Source: CAD feature listing. Evaluate the final solid. Frame: model axes, mm. A direction names the side the tool comes from. Round coordinates to 2 decimals unless told otherwise and drop trailing zeros. Order: outer loops, then holes, each group sorted by start corner. A loop starts at its lowest first (then second) coordinate and runs counter-clockwise, first axis right, second up. Notation, with made-up numbers: (25, 57.5) -> (51, 57.5) arc R21 cw to (51, 68.5) -> close; hole circle Ø1 at (-37, 50.5). An arc over 180 degrees is marked (long way). Answer as CSV lines item,"result".
from build123d import *

# Parameters (mm, degrees)
CYLINDER081_R     = 1.6
CYLINDER081_DEPTH = 1.5
CYLINDER082_R     = 4
CYLINDER082_DEPTH = 1.5
CYLINDER083_R     = 1.6
CYLINDER083_DEPTH = 1.5
CYLINDER084_R     = 4
CYLINDER084_DEPTH = 1.5
BOX207_W          = 14
BOX207_H          = 9
BOX207_DEPTH      = 1.5
BOX206_W          = 14
BOX206_H          = 9
BOX206_DEPTH      = 1.5
BOX205_W          = 36
BOX205_H          = 12
BOX205_DEPTH      = 1.5
FILLET050_R       = 2
CYLINDER080_R     = 1.6
CYLINDER080_DEPTH = 1.5
CYLINDER079_R     = 4
CYLINDER079_DEPTH = 1.5


with BuildPart() as cylinder162:
    # Cylinder081 → Cylinder081 (new body)
    with BuildSketch(Plane(origin=(70.25, 15, 8.3), x_dir=(1, 0, 0), z_dir=(0, 0, 1))):
        Circle(CYLINDER081_R)
    extrude(amount=CYLINDER081_DEPTH)


with BuildPart() as cut104:
    # Cylinder082 → Cylinder082 (new body)
    with BuildSketch(Plane(origin=(70.25, 15, 8.3), x_dir=(1, 0, 0), z_dir=(0, 0, 1))):
        Circle(CYLINDER082_R)
    extrude(amount=CYLINDER082_DEPTH)

    # Cut104: cut Cylinder162
    add(cylinder162.part, mode=Mode.SUBTRACT)


with BuildPart() as cylinder164:
    # Cylinder083 → Cylinder083 (new body)
    with BuildSketch(Plane(origin=(59.25, 32.25, 8.3), x_dir=(1, 0, 0), z_dir=(0, 0, 1))):
        Circle(CYLINDER083_R)
    extrude(amount=CYLINDER083_DEPTH)


with BuildPart() as cut105:
    # Cylinder084 → Cylinder084 (new body)
    with BuildSketch(Plane(origin=(59.25, 32.25, 8.3), x_dir=(1, 0, 0), z_dir=(0, 0, 1))):
        Circle(CYLINDER084_R)
    extrude(amount=CYLINDER084_DEPTH)

    # Cut105: cut Cylinder164
    add(cylinder164.part, mode=Mode.SUBTRACT)


with BuildPart() as cube196:
    # Box207 → Box207 (new body)
    with BuildSketch(Plane(origin=(61, 19.5, 8.3), x_dir=(1, 0, 0), z_dir=(0, 0, 1))):
        with Locations((7, 4.5)):
            Rectangle(BOX207_W, BOX207_H)
    extrude(amount=BOX207_DEPTH)


with BuildPart() as cube195:
    # Box206 → Box206 (new body)
    with BuildSketch(Plane(origin=(43.5, 19.5, 8.3), x_dir=(1, 0, 0), z_dir=(0, 0, 1))):
        with Locations((7, 4.5)):
            Rectangle(BOX206_W, BOX206_H)
    extrude(amount=BOX206_DEPTH)


with BuildPart() as fillet050:
    # Box205 → Box205 (new body)
    with BuildSketch(Plane(origin=(41, 18, 8.3), x_dir=(1, 0, 0), z_dir=(0, 0, 1))):
        with Locations((18, 6)):
            Rectangle(BOX205_W, BOX205_H)
    extrude(amount=BOX205_DEPTH)

    # Cut106: cut Cube195
    add(cube195.part, mode=Mode.SUBTRACT)

    # Cut107: cut Cube196
    add(cube196.part, mode=Mode.SUBTRACT)

    # Fillet050
    fillet050_edges = [fillet050.edges().sort_by_distance(p)[0] for p in [
        (41, 18, 9.05),
        (41, 30, 9.05),
        (77, 18, 9.05),
        (77, 30, 9.05),
    ]]
    fillet(fillet050_edges, radius=FILLET050_R)


with BuildPart() as cylinder161:
    # Cylinder080 → Cylinder080 (new body)
    with BuildSketch(Plane(origin=(47.75, 15, 8.3), x_dir=(1, 0, 0), z_dir=(0, 0, 1))):
        Circle(CYLINDER080_R)
    extrude(amount=CYLINDER080_DEPTH)


with BuildPart() as fusion064:
    # Cylinder079 → Cylinder079 (new body)
    with BuildSketch(Plane(origin=(47.75, 15, 8.3), x_dir=(1, 0, 0), z_dir=(0, 0, 1))):
        Circle(CYLINDER079_R)
    extrude(amount=CYLINDER079_DEPTH)

    # Cut103: cut Cylinder161
    add(cylinder161.part, mode=Mode.SUBTRACT)

    # Fusion064: union Cut104, Cut105, Fillet050
    add(cut104.part)
    add(cut105.part)
    add(fillet050.part)


solid = fusion064.part
1. Pin query (flat end, axial travel): pin 1 (0.8 mm diameter, centred on x = 68.5, z = 9, fed in from +Y). Return the tip coordinate at first contact, or that it passes through.
Results below:
pin 1,"y = 30"
2. Reachability of faces 1 (the flat face through (43.5, 24, 9)), 2 (the flat face through (41, 24, 9)) from +Z, -Z, +X, -X, +Y, -Y: full face, straight path, thin tool, end or side. Return the list, or none.
Results below:
face 1,"+Z, -Z"
face 2,"+Z, -Z, -X, +Y, -Y"
3. Line query: L1, parallel to X at y = 26.5, z = 9.1; L2, parallel to Y at x = 65, z = 8.75; L3, parallel to Y at x = 59.25, z = 9.55. Output: solid intervals per line, ascending. Write a range as [from, to].
Results below:
L1,"[41, 43.5], [57.5, 61], [75, 77]"
L2,"[18, 19.5], [28.5, 30]"
L3,"[18, 30.65], [33.85, 36.25]"
4. Section query B-B on y = 26. Return loops of the section in (x, z).
Results below:
outline,"(41, 8.3) -> (43.5, 8.3) -> (43.5, 9.8) -> (41, 9.8) -> close; (57.5, 8.3) -> (61, 8.3) -> (61, 9.8) -> (57.5, 9.8) -> close; (75, 8.3) -> (77, 8.3) -> (77, 9.8) -> (75, 9.8) -> close"
5. Section query C-C on y = 15. Return loops of the section in (x, z), and give its area (3 significant figures).
Results below:
outline,"(43.75, 8.3) -> (46.15, 8.3) -> (46.15, 9.8) -> (43.75, 9.8) -> close; (49.35, 8.3) -> (51.75, 8.3) -> (51.75, 9.8) -> (49.35, 9.8) -> close; (66.25, 8.3) -> (68.65, 8.3) -> (68.65, 9.8) -> (66.25, 9.8) -> close; (71.85, 8.3) -> (74.25, 8.3) -> (74.25, 9.8) -> (71.85, 9.8) -> close"
area,"14.4 mm2"
6. Mould query, pull axis X, two halves, no side actions, for faces 3 (the flat face through (61, 24, 9)), 4 (the cylindrical face through (76.4, 18.57, 9.06)), 5 (the flat face through (59, 24, 8.3)). Classes: released by +X, released by -X, zero draft, split by the parting line, or undercut.
Results below:
face 3,"undercut"
face 4,"released by +X"
face 5,"zero draft"
7. Section query D-D on z = 8.75. Return loops of the section in (x, y).
Results below:
outline,"(41, 20) arc R2 ccw to (43, 18) -> (45.1, 18) arc R4 ccw (long way) to (50.4, 18) -> (67.6, 18) arc R4 ccw (long way) to (72.9, 18) -> (75, 18) arc R2 ccw to (77, 20) -> (77, 28) arc R2 ccw to (75, 30) -> (62.56, 30) arc R4 ccw (long way) to (55.94, 30) -> (43, 30) arc R2 ccw to (41, 28) -> close; hole (43.5, 19.5) -> (57.5, 19.5) -> (57.5, 28.5) -> (43.5, 28.5) -> close; hole circle Ø3.2 at (47.75, 15); hole circle Ø3.2 at (59.25, 32.25); hole (61, 19.5) -> (75, 19.5) -> (75, 28.5) -> (61, 28.5) -> close; hole circle Ø3.2 at (70.25, 15)"
8. Section query A-A on x = 47.75. Return loops of the section in (y, z).
Results below:
outline,"(11, 8.3) -> (13.4, 8.3) -> (13.4, 9.8) -> (11, 9.8) -> close; (16.6, 8.3) -> (19.5, 8.3) -> (19.5, 9.8) -> (16.6, 9.8) -> close; (28.5, 8.3) -> (30, 8.3) -> (30, 9.8) -> (28.5, 9.8) -> close"
